Work out the finished part from the listing and answer in its coordinate system (mm). A direction names the side the tool comes from. Coordinates: 2 decimals unless noted, no trailing zeros. Write each loop counter-clockwise with the first axis right and the second up, starting at its lowest first coordinate (ties: lowest second). Pieces come first, ordered by that corner, then holes. Notation, with made-up numbers: M 20,-2 L 27,-2 A21 ccw 27,7 Z; hole C 51.5,64.5 d8. An arc over 180 degrees is marked long. Use CSV: the item, a comma, the result in double quotes.
from build123d import *

# Parameters (mm, degrees)
SKETCH_1_R                = 22
EXTRUDE_1_DEPTH           = 2
SKETCH_3_R                = 1.5
CUT_EXTRUDE_1_DEPTH       = 3
SKETCH_4_R                = 3.5
CUT_EXTRUDE_2_DEPTH       = 3
SKETCH_6_R                = 3
EXTRUDE_3_DEPTH           = 10.5
SKETCH_8_R                = 1.25
CUT_EXTRUDE_4_DEPTH       = 12.5
CUT_EXTRUDE_3_DEPTH       = 6
PATTERN_CIRCULAR_1_COUNT  = 4
FILLET_2_R                = 1.5
FILLET_3_R                = 1.5
PATTERN_CIRCULAR_2_COUNT  = 2
REVOLVE_1_ANGLE           = 125
REVOLVE_1_OTHER_WAY_ANGLE = 125


with BuildPart() as part:
    # 草图1 → 凸台-拉伸1 (new body)
    with BuildSketch(Plane.XY):
        Circle(SKETCH_1_R)
    extrude(amount=EXTRUDE_1_DEPTH)

    # 草图3 → 切除-拉伸1 (cut)
    with BuildSketch(Plane(origin=(0, 0, 0), x_dir=(-1, 0, 0), z_dir=(0, 0, -1))):
        with Locations((9.5, 0)):
            Circle(SKETCH_3_R)
        with Locations((0, 8)):
            Circle(SKETCH_3_R)
    cut_extrude_1 = extrude(amount=-CUT_EXTRUDE_1_DEPTH, mode=Mode.SUBTRACT)

    # 草图4 → 切除-拉伸2 (cut)
    with BuildSketch(Plane(origin=(0, 0, 0), x_dir=(-1, 0, 0), z_dir=(0, 0, -1))):
        Circle(SKETCH_4_R)
    extrude(amount=-CUT_EXTRUDE_2_DEPTH, mode=Mode.SUBTRACT)

    # 草图6 → 凸台-拉伸3 (add)
    with BuildSketch(Plane(origin=(0, 0, 0), x_dir=(-1, 0, 0), z_dir=(0, 0, -1))):
        with Locations((0, -19)):
            Circle(SKETCH_6_R)
    extrude_3 = extrude(amount=EXTRUDE_3_DEPTH)

    # 草图8 → 切除-拉伸4 (cut)
    with BuildSketch(Plane(origin=(0, 0, -10.5), x_dir=(-1, 0, 0), z_dir=(0, 0, -1))):
        with Locations((0, -19)):
            Circle(SKETCH_8_R)
    cut_extrude_4 = extrude(amount=-CUT_EXTRUDE_4_DEPTH, mode=Mode.SUBTRACT)

    # 草图7 → 切除-拉伸3 (cut)
    with BuildSketch(Plane(origin=(0, 0, 0), x_dir=(-1, 0, 0), z_dir=(0, 0, -1))):
        Polygon((-2.572740594, 10.290962376), (-10.290962376, 2.572740594), (-30.512752563, 7.628188141), (-7.628188141, 30.512752563), align=None)
    cut_extrude_3 = extrude(amount=-CUT_EXTRUDE_3_DEPTH, mode=Mode.SUBTRACT)

    # 阵列(圆周)1: 凸台-拉伸3, 切除-拉伸4, 切除-拉伸3 ×4 about axis
    pattern_circular_1_axis = Axis((0, 0, 0), (0, 0, 1))
    for i in range(1, PATTERN_CIRCULAR_1_COUNT):
        add(extrude_3.rotate(pattern_circular_1_axis, i * 360 / PATTERN_CIRCULAR_1_COUNT))
        add(cut_extrude_4.rotate(pattern_circular_1_axis, i * 360 / PATTERN_CIRCULAR_1_COUNT), mode=Mode.SUBTRACT)
        add(cut_extrude_3.rotate(pattern_circular_1_axis, i * 360 / PATTERN_CIRCULAR_1_COUNT), mode=Mode.SUBTRACT)

    # 圆角2
    fillet_2_edges = [part.edges().sort_by_distance(p)[0] for p in [
        (21.343135003, -5.335783751, 1),
        (5.335783751, -21.343135003, 1),
        (5.335783751, 21.343135003, 1),
        (21.343135003, 5.335783751, 1),
        (-21.343135003, 5.335783751, 1),
        (-5.335783751, 21.343135003, 1),
        (-5.335783751, -21.343135003, 1),
        (-21.343135003, -5.335783751, 1),
    ]]
    fillet(fillet_2_edges, radius=FILLET_2_R)

    # 圆角3
    fillet_3_edges = [part.edges().sort_by_distance(p)[0] for p in [
        (2.572740594, -10.290962376, 1),
        (10.290962376, -2.572740594, 1),
        (10.290962376, 2.572740594, 1),
        (2.572740594, 10.290962376, 1),
        (-2.572740594, 10.290962376, 1),
        (-10.290962376, 2.572740594, 1),
        (-10.290962376, -2.572740594, 1),
        (-2.572740594, -10.290962376, 1),
    ]]
    fillet(fillet_3_edges, radius=FILLET_3_R)

    # 阵列(圆周)2: 切除-拉伸1 ×2 about axis
    pattern_circular_2_axis = Axis((0, 0, 0), (0, 0, 1))
    for i in range(1, PATTERN_CIRCULAR_2_COUNT):
        add(cut_extrude_1.rotate(pattern_circular_2_axis, i * 360 / PATTERN_CIRCULAR_2_COUNT), mode=Mode.SUBTRACT)

    # 草图10 → 旋转1 (revolve)
    with BuildSketch(Plane(origin=(0, 0, 0), x_dir=(0, 0, -1), z_dir=(1, 0, 0))):
        Polygon((0, -16.312681485), (0, -14.5), (3.69057161, -16.312681485), align=None)
    revolve(axis=Axis((0, -19, 2), (0, 0, -1)), revolution_arc=REVOLVE_1_ANGLE)

    # 草图10 → 旋转1 other way (revolve)
    with BuildSketch(Plane(origin=(0, 0, 0), x_dir=(0, 0, -1), z_dir=(1, 0, 0))):
        Polygon((0, -16.312681485), (0, -14.5), (3.69057161, -16.312681485), align=None)
    revolve(axis=Axis((0, -19, 2), (0, 0, 1)), revolution_arc=REVOLVE_1_OTHER_WAY_ANGLE)


solid = part.part
Item 1: Given pin 1 (6 mm diameter, centred on y = 4, z = -1.5, fed in from +X); pin 2 (2 mm diameter, centred on x = 19, y = 0, fed in from +Z); pin 3 (4 mm diameter, centred on x = -9.5, y = 0, fed in from +Z); pin 4 (3 mm diameter, centred on y = -17, z = -2.5, fed in from -X), each flat-ended and moving along its own axis, determine where each tip first touches the part or whether it passes through.
Answer:
pin 1,"stops at x = 21.96"
pin 2,"passes through"
pin 3,"stops at z = 2"
pin 4,"stops at x = -3.71"
Item 2: A tool of negligible diameter and unlimited length cuts with its end or side. For faces 4 (the face through (6.477, -6.386, 0.986)), 5 (the face through (-16, 4, 1)), 6 (the face through (2.81, -20.97, -0.87)), 7 (the face through (-21.93, -0.65, -5.18)), from which of +Z, -Z, +X, -X, +Y, -Y can it reach the whole face along a straight path? Write none if from no direction.
Answer:
face 4,"+Z, -Z"
face 5,"+Z, -Z, +Y"
face 6,"-Z, -Y"
face 7,"-Z"
Item 3: The part is cut by section D-D (y = 8). Write down the section's boundary in (x, z).
Answer:
outline,"M -4.86,0 L -1.5,0 L -1.5,2 L -4.86,2 Z; M 1.5,0 L 4.86,0 L 4.86,2 L 1.5,2 Z"
Item 4: The part is cut by section B-B (x = -9). Write down the section's boundary in (y, z), then the cut area to 3 significant figures.
Answer:
outline,"M -3.86,0 L -1.41,0 L -1.41,2 L -3.86,2 Z; M 1.41,0 L 3.86,0 L 3.86,2 L 1.41,2 Z"
area,"9.80 mm2"
Item 5: Consider probe 1 along Y at (x, z) = (0, 1); probe 2 along Y at (x, z) = (0, -8). Determine where each line is inside the solid, lowest interval first.
Answer:
probe 1,"y = -22 to -20.25, -17.75 to -9.5, -6.5 to -3.5, 3.5 to 6.5, 9.5 to 17.75, 20.25 to 22"
probe 2,"y = -22 to -20.25, -17.75 to -16, 16 to 17.75, 20.25 to 22"
Item 6: The part is cut by section C-C (z = 1.25). Count the separate pieces of the cut face and the enclosed holes in it, then the cut area to 3 significant figures.
Answer:
separate pieces,"1"
enclosed holes,"9"
area,"583 mm2"
Item 7: The part is cut by section A-A (y = -19). Write down the section's boundary in (x, z).
Answer:
outline,"M -4.75,0 L -4.5,0 L -3,-3.05 L -3,-10.5 L -1.25,-10.5 L -1.25,2 L -4.75,2 Z; M 1.25,-10.5 L 3,-10.5 L 3,-3.05 L 4.5,0 L 4.75,0 L 4.75,2 L 1.25,2 Z"
Item 8: For a pull along X with two mould halves and no side action, classify faces 1 (the face through (-20, 1, -10.5)), 2 (the face through (-20.22, -0.27, -4.34)), 3 (the face through (-4, -16, 1)) as released by +X, released by -X, zero draft, split by the parting line, or undercut.
Answer:
face 1,"zero draft"
face 2,"undercut"
face 3,"released by -X"
